Check sheet for the modelled part. Datum: model origin and axes. Units: mm. A direction names the side the tool comes from. Coordinates: 2 decimals unless noted, no trailing zeros. Write each loop counter-clockwise with the first axis right and the second up, starting at its lowest first coordinate (ties: lowest second). Pieces come first, ordered by that corner, then holes. Notation, with made-up numbers: (15.25, -21.5) - (28.25, -21.5) arc R9 cw to (28.25, -5.5) - close; hole circle Ø2 at (-30, 86.25). An arc over 180 degrees is marked (long way). Use one line per item in the form item = value. Start each with the question number.
1. Cross-section at B-B on z = 7. Record the boundary of the cut face in (x, y), then the cut area to 3 significant figures.
2. Go/stop test with flat-tipped pins: pin 1 Ø2 at (x, z) = (-30, 13) entering from -Y; pin 2 Ø1.5 at (y, z) = (29, 8.5) entering from -X; pin 3 Ø2.5 at (x, y) = (0, 0) entering from -Z; pin 4 Ø12 at (x, y) = (-3, 26) entering from -Z. Record where each tip stops, or that it passes through.
3. Scan lines: line 1 along Y through (x, z) = (0, 7.65); line 2 along Z through (x, y) = (29, 15.5); line 3 along X through (y, z) = (-2, 9). Record each from-to range of solid material in increasing order.
4. Draft check along Z on faces 4 (the face through (8, 1, 0)), 5 (the face through (-30.235, -23.183, 7.395)), 6 (the face through (-7.18, -32.31, 7.46)). Enter one of: +Z half, -Z half, draft (parallel to the pull), parting line (faces both ways), or undercut.
5. Tool access check on faces 1 (the face through (7, 0, 10)), 2 (the face through (0, 0, 10)), 3 (the face through (-1, 1, 15)). Record the directions out of +Z, -Z, +X, -X, +Y, -Y that give a thin tool (end or side, any length) a straight path to the whole face; none if there is none.
6. Cross-section at A-A on y = 0. Record the boundary of the cut face in (x, z), then the cut area to 3 significant figures.
7. Cross-section at D-D on x = -24. Record the boundary of the cut face in (y, z), then the cut area to 3 significant figures.
```python
from build123d import *

# Parameters (mm, degrees)
SKETCH1_R                       = 38.1
BOSS_EXTRUDE1_DEPTH             = 15
F_3_0MM_CLEARANCE_DOWEL_HOLE1_D = 3
SHELL3_T                        = -5
BOSS_EXTRUDE2_START             = 10
SKETCH1_2_R                     = 38.1
BOSS_EXTRUDE2_DEPTH             = 5


with BuildPart() as part:
    # Sketch1 → Boss-Extrude1 (new body)
    with BuildSketch(Plane.XY):
        Circle(SKETCH1_R)
    extrude(amount=BOSS_EXTRUDE1_DEPTH)

    # Ø3.0mm Clearance Dowel Hole1 (through all)
    with Locations(Plane.XY.offset(15)):
        with Locations((0, 0)):
            Hole(F_3_0MM_CLEARANCE_DOWEL_HOLE1_D / 2)

    # Shell3
    shell3_openings = [part.faces().sort_by_distance(p)[0] for p in [
        (-37.022369265, 0, 15),
    ]]
    offset(amount=SHELL3_T, openings=shell3_openings, kind=Kind.INTERSECTION)

    # Sketch1<2> → Boss-Extrude2 (add)
    with BuildSketch(Plane.XY.offset(BOSS_EXTRUDE2_START)):
        Circle(SKETCH1_2_R)
    extrude(amount=BOSS_EXTRUDE2_DEPTH)


solid = part.part
```
Final values:
q1.outline = circle Ø76.2 at (0, 0); circle Ø13 at (0, 0); hole circle Ø66.2 at (0, 0); hole circle Ø3 at (0, 0)
q1.area = 1,240 mm²
q2.pin_1 = -24.71
q2.pin_2 = -25.56
q2.pin_3 = 10
q2.pin_4 = 0
q3.line_1 = -38.1 to -33.1, -6.5 to -1.5, 1.5 to 6.5, 33.1 to 38.1
q3.line_2 = 0 to 5, 10 to 15
q3.line_3 = -38.05 to -33.04, -6.18 to 6.18, 33.04 to 38.05
q4.face_4 = -Z half
q4.face_5 = draft
q4.face_6 = undercut
q5.face_1 = none
q5.face_2 = -Z
q5.face_3 = +Z, +X, -X, +Y, -Y
q6.outline = (-38.1, 0) - (-1.5, 0) - (-1.5, 10) - (1.5, 10) - (1.5, 0) - (38.1, 0) - (38.1, 15) - (-38.1, 15) - close; hole (-33.1, 5) - (-6.5, 5) - (-6.5, 10) - (-33.1, 10) - close; hole (6.5, 5) - (33.1, 5) - (33.1, 10) - (6.5, 10) - close
q6.area = 847 mm²
q7.outline = (-29.59, 0) - (29.59, 0) - (29.59, 15) - (-29.59, 15) - close; hole (-22.79, 5) - (22.79, 5) - (22.79, 10) - (-22.79, 10) - close
q7.area = 660 mm²
